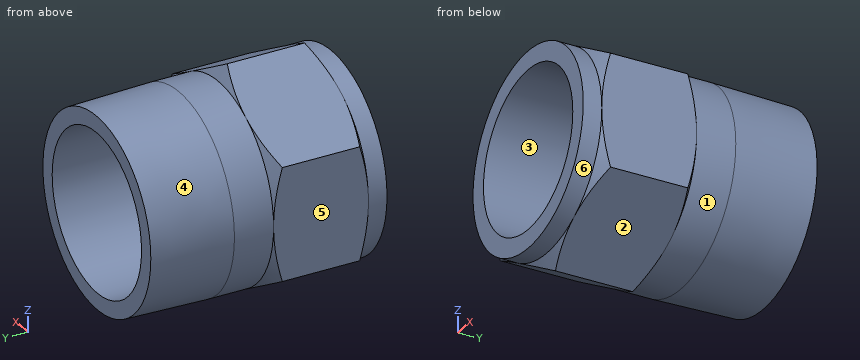
from build123d import *

# Parameters (mm, degrees)
SKETCH2_R           = 19.25
BOSS_EXTRUDE1_DEPTH = 57


with BuildPart() as part:
    # Sketch2 → Boss-Extrude1 (new body)
    with BuildSketch(Plane(origin=(0, 0, 0), x_dir=(1, 0, 0), z_dir=(0, 1, 0))):
        Polygon((0, 27.424137787), (-23.75, 13.712068893), (-23.75, -13.712068893), (0, -27.424137787), (23.75, -13.712068893), (23.75, 13.712068893), align=None)
        Circle(SKETCH2_R, mode=Mode.SUBTRACT)
    extrude(amount=BOSS_EXTRUDE1_DEPTH)

    # Sketch3 → Cut-Revolve2 (revolve, cut)
    with BuildSketch(Plane.XY):
        Polygon((0, 57), (-23.25, 57), (-23.75, 37), (-23.75, 27.5), (-33.75, 21.726497308), (-33.75, 10.273502692), (-23.75, 4.5), (-23.75, 0), (-45.690595107, 0), (-45.690595107, 61.224990586), (0, 61.224990586), align=None)
    revolve(axis=Axis((0, 64.286240116, 0), (0, -1, 0)), mode=Mode.SUBTRACT)


solid = part.part
Source: CAD feature listing. Evaluate the final solid. Frame: model axes, mm. Face numbers are marked on the shaded views. A direction names the side the tool comes from. Give positions to 0.01 mm unless a question says otherwise; leave off trailing zeros. Write each loop counter-clockwise with the first axis right and the second up, starting at its lowest first coordinate (ties: lowest second). Pieces come first, ordered by that corner, then holes. Notation, with made-up numbers: M -30,69.5 L 5,69.5 A29 ccw 5,94.5 Z; hole C 47.5,63 d11. An arc over 180 degrees is marked long. Return JSON: item names as keys, results as strings. Group by question number.
1) Ray query, L1, parallel to X at y = 13, z = 0; L2, parallel to Z at x = -14, y = 9. Return the intervals inside material, ascending.
2) Cut plane B-B, the plane y = 46. Output: boundary loops of the cut face in (x, z) (3 decimals).
3) Cut plane A-A, the plane y = 13.5. Output: boundary loops of the cut face in (x, z), then the cut area to 3 significant figures.
4) Set-up query: the marked faces 4, 5 and 6. Return all of +Z, -Z, +X, -X, +Y, -Y with unobstructed straight access to the full face (end or side cutting, diameter ignored); none if empty.
5) First-contact query: pin 1 Ø5 at (y, z) = (42.5, -19) entering from +X; pin 2 Ø12 at (y, z) = (34, 10.5) entering from +X; pin 3 Ø12 at (y, z) = (46.5, -18.5) entering from +X; pin 4 Ø12 at (x, z) = (-12.5, -17) entering from -Y. Flat tips, straight axial feed; report the tip coordinate or a pass-through.
6) Draft query along Z for the marked faces 1, 2 and 3. Return one class per face: released by +Z, released by -Z, zero draft, split by the parting line, or undercut.
Data:
{
 "1": {"L1": "x = -23.75 to -19.25, 19.25 to 23.75", "L2": "z = -19.34 to -13.21, 13.21 to 19.34"},
 "2": {"outline": "C 0,0 d47.05; hole C 0,0 d38.5"},
 "3": {"outline": "M -23.75,-13.71 L 0,-27.42 L 23.75,-13.71 L 23.75,13.71 L 0,27.42 L -23.75,13.71 Z; hole C 0,0 d38.5", "area": "790 mm²"},
 "4": {"face 4": "+Y", "face 5": "+Z, -Z, -X, +Y, -Y", "face 6": "-Y"},
 "5": {"pin 1": "stops at x = 16.89", "pin 2": "stops at x = 23.32", "pin 3": "stops at x = 19.92", "pin 4": "stops at y = 0"},
 "6": {"face 1": "split by the parting line", "face 2": "released by -Z", "face 3": "undercut"}
}
